Here's how the part is built. I have some questions about the finished solid (model axes, mm). A direction names the side the tool comes from. Coordinates: 2 decimals unless noted, no trailing zeros. Write each loop counter-clockwise with the first axis right and the second up, starting at its lowest first coordinate (ties: lowest second). Pieces come first, ordered by that corner, then holes.
Item 1: I'm going to push flat-ended pins straight in: P1, Ø3, axis at x = 13.97, z = -13.97, coming from the +Y side; P2, Ø10, axis at y = 16, z = -85, coming from the -X side; P3, Ø1, axis at y = 14.5, z = -32, coming from the -X side; P4, Ø5, axis at x = 14.5, z = -33.5, coming from the +Y side. Where does each tip first touch, or does it pass through?
Item 2: I want a section at B-B (z = -54). Please give me the cut outline in (x, y) (3 decimals).
Item 3: If we mould it in two halves opening along Z, with no side actions, what happens to faces 1 (the face through (9, 8, 0)), 2 (the face through (10, 0, -53)), 3 (the face through (6, 17, -81.661))? For each: pulls with the +Z half, pulls with the -Z half, needs draft (parallel to the pull), parting line crosses it, or undercut.
Item 4: Please list where these lines run through material, in increasing order: line 1 (Z direction, x = 13.97, y = 1.75); line 2 (X direction, y = 7.25, z = -96); line 3 (Y direction, x = 8.5, z = -78).
Item 5: I want a section at A-A (z = -13.97). Please give me the cut outline in (x, y) (3 decimals), and give its area (3 significant figures).
Item 6: For faces 4 (the face through (15, 2, -82.55)), 5 (the face through (7, 11.43, -111)), 6 (the face through (15, 3.048, -42)), 7 (the face through (1.29, 10.18, -110.81)), which set-ups out of +Z, -Z, +X, -X, +Y, -Y let a thin tool reach every point of the face, with its end or its side?
from build123d import *

# Parameters (mm, degrees)
SKETCH1_W           = 77.47
SKETCH1_H           = 133.35
BOSS_EXTRUDE1_DEPTH = 11.43
SKETCH2_R           = 3.429
CUT_EXTRUDE1_DEPTH  = 134.35
CUT_EXTRUDE2_DEPTH  = 12.43
SKETCH4_W           = 54.61
SKETCH4_H           = 6.35
CUT_EXTRUDE3_DEPTH  = 134.35
CHAMFER1_SIZE       = 2.54
CUT_EXTRUDE4_DEPTH  = 12.43
SKETCH6_W           = 53.34
SKETCH6_H           = 82.55
CUT_EXTRUDE5_DEPTH  = 12.43
SKETCH7_R           = 1.778
HOLE_CUTS_1_DEPTH   = 6.08
BOSS_EXTRUDE5_DEPTH = 88.9
SKETCH18_W          = 6.35
SKETCH18_H          = 5.08
CUT_EXTRUDE13_DEPTH = 76.2
HOLE_CUTS_2_REACH   = 10.608
SKETCH19_R          = 1.778
SKETCH20_W          = 88.9
SKETCH20_H          = 11.176
CUT_EXTRUDE16_DEPTH = 1.27
CUT_EXTRUDE22_DEPTH = 134.35
SKETCH22_W          = 6.35
SKETCH22_H          = 82.55
CUT_EXTRUDE18_DEPTH = 2.032
SKETCH23_W          = 1.676805636
SKETCH23_H          = 88.9
BOSS_EXTRUDE6_DEPTH = 1.27
CUT_EXTRUDE19_REACH = 10.019
SKETCH24_W          = 69.85
SKETCH24_H          = 9.3345
CUT_EXTRUDE20_REACH = 12.28
SKETCH25_W          = 1.27
SKETCH25_H          = 88.9
CUT_EXTRUDE21_REACH = 7.08
SKETCH26_W          = 6.35
SKETCH26_H          = 6.35


with BuildPart() as part:
    # Sketch1 → Boss-Extrude1 (new body)
    with BuildSketch(Plane(origin=(0, 0, 0), x_dir=(1, 0, 0), z_dir=(0, 1, 0))):
        with Locations((38.735, 66.675)):
            Rectangle(SKETCH1_W, SKETCH1_H)
    extrude(amount=BOSS_EXTRUDE1_DEPTH)

    # Sketch2 → Cut-Extrude1 (cut, through all)
    with BuildSketch(Plane.XY):
        with Locations((5.715, 5.715)):
            Circle(SKETCH2_R)
        with Locations((71.755, 5.715)):
            Circle(SKETCH2_R)
    extrude(amount=-CUT_EXTRUDE1_DEPTH, mode=Mode.SUBTRACT)

    # Sketch3 → Cut-Extrude2 (cut, through all)
    with BuildSketch(Plane(origin=(0, 11.43, 0), x_dir=(1, 0, 0), z_dir=(0, 1, 0))):
        with BuildLine():
            Line((11.43, 133.35), (11.43, 95.25))
            ThreePointArc((11.43, 95.25), (15.149743879, 86.269743879), (24.13, 82.55))
            Line((24.13, 82.55), (53.34, 82.55))
            ThreePointArc((53.34, 82.55), (62.320256121, 86.269743879), (66.04, 95.25))
            Line((66.04, 95.25), (66.04, 133.35))
            Line((66.04, 133.35), (11.43, 133.35))
        make_face()
    extrude(amount=-CUT_EXTRUDE2_DEPTH, mode=Mode.SUBTRACT)

    # Sketch4 → Cut-Extrude3 (cut, through all)
    with BuildSketch(Plane(origin=(0, 0, -133.35), x_dir=(-1, 0, 0), z_dir=(0, 0, -1))):
        with Locations((-38.735, 8.255)):
            Rectangle(SKETCH4_W, SKETCH4_H)
    extrude(amount=-CUT_EXTRUDE3_DEPTH, mode=Mode.SUBTRACT)

    # Chamfer1
    chamfer1_edges = [part.edges().sort_by_distance(p)[0] for p in [
        (77.47, 11.43, -66.675),
        (0, 11.43, -66.675),
        (77.47, 0, -66.675),
        (0, 0, -66.675),
    ]]
    chamfer(chamfer1_edges, length=CHAMFER1_SIZE)

    # Sketch5 → Cut-Extrude4 (cut, through all)
    with BuildSketch(Plane(origin=(0, 11.43, 0), x_dir=(1, 0, 0), z_dir=(0, 1, 0))):
        Polygon((11.43, 95.25), (11.43, 82.55), (77.47, 82.55), (77.47, 133.35), (11.43, 133.35), align=None)
    extrude(amount=-CUT_EXTRUDE4_DEPTH, mode=Mode.SUBTRACT)

    # Sketch6 → Cut-Extrude5 (cut, through all)
    with BuildSketch(Plane(origin=(0, 11.43, 0), x_dir=(1, 0, 0), z_dir=(0, 1, 0))):
        with Locations((50.8, 41.275)):
            Rectangle(SKETCH6_W, SKETCH6_H)
    extrude(amount=-CUT_EXTRUDE5_DEPTH, mode=Mode.SUBTRACT)

    # Sketch7 → Hole Cuts 1 (cut, through all)
    with BuildSketch(Plane(origin=(0, 5.08, 0), x_dir=(1, 0, 0), z_dir=(0, 1, 0))):
        with Locations((13.97, 74.93)):
            Circle(SKETCH7_R)
        with Locations((13.97, 13.97)):
            Circle(SKETCH7_R)
    extrude(amount=-HOLE_CUTS_1_DEPTH, mode=Mode.SUBTRACT)

    # Sketch17 → Boss-Extrude5 (add)
    with BuildSketch(Plane.XY):
        Polygon((0, 8.89), (0, 11.869940905), (5.588, 21.548640818), (8.851738686, 19.664320409), (5.930738686, 14.605), (11.43, 11.43), (2.54, 11.43), align=None)
    extrude(amount=-BOSS_EXTRUDE5_DEPTH)

    # Sketch18 → Cut-Extrude13 (cut)
    with BuildSketch(Plane.XY):
        with Locations((20.955, 2.54)):
            Rectangle(SKETCH18_W, SKETCH18_H)
    extrude(amount=-CUT_EXTRUDE13_DEPTH, mode=Mode.SUBTRACT)

    # Sketch19 → Hole Cuts 2 (cut, up to next)
    with BuildSketch(Plane(origin=(-1.876096497, 1.083164817, 0), x_dir=(0, 0, -1), z_dir=(0.866025404, -0.5, 0)), mode=Mode.PRIVATE) as hole_cuts_2_sk1:
        with Locations((8.382, 19.423670365)):
            Circle(SKETCH19_R)
    hole_cuts_2_tool1 = extrude(hole_cuts_2_sk1.sketch, amount=-HOLE_CUTS_2_REACH, mode=Mode.PRIVATE) & part.part
    add(hole_cuts_2_tool1.solids().sort_by_distance((7.835739, 17.904557, -8.382))[0], mode=Mode.SUBTRACT)
    # Sketch19 → Hole Cuts 2 (cut, up to next)
    with BuildSketch(Plane(origin=(-1.876096497, 1.083164817, 0), x_dir=(0, 0, -1), z_dir=(0.866025404, -0.5, 0)), mode=Mode.PRIVATE) as hole_cuts_2_sk2:
        with Locations((85.09, 19.423670365)):
            Circle(SKETCH19_R)
    hole_cuts_2_tool2 = extrude(hole_cuts_2_sk2.sketch, amount=-HOLE_CUTS_2_REACH, mode=Mode.PRIVATE) & part.part
    add(hole_cuts_2_tool2.solids().sort_by_distance((7.835739, 17.904557, -85.09))[0], mode=Mode.SUBTRACT)

    # Sketch20 → Cut-Extrude16 (cut)
    with BuildSketch(Plane(origin=(-5.139835183, 2.967485226, 0), x_dir=(0, 0, 1), z_dir=(-0.866025404, 0.5, 0))):
        with Locations((-44.45, 15.867670365)):
            Rectangle(SKETCH20_W, SKETCH20_H)
    extrude(amount=-CUT_EXTRUDE16_DEPTH, mode=Mode.SUBTRACT)

    # Sketch31 → Cut-Extrude22 (cut, through all)
    with BuildSketch(Plane.XY):
        Polygon((8.14000854, 20.075238), (12.539417591, 17.535238), (9.618417591, 12.475917591), (5.21900854, 15.015917591), align=None)
    extrude(amount=-CUT_EXTRUDE22_DEPTH, mode=Mode.SUBTRACT)

    # Sketch22 → Cut-Extrude18 (cut)
    with BuildSketch(Plane(origin=(0, 5.08, 0), x_dir=(1, 0, 0), z_dir=(0, 1, 0))):
        with Locations((14.605, 41.275)):
            Rectangle(SKETCH22_W, SKETCH22_H)
    extrude(amount=-CUT_EXTRUDE18_DEPTH, mode=Mode.SUBTRACT)

    # Sketch23 → Boss-Extrude6 (add)
    with BuildSketch(Plane(origin=(10.727835183, 18.581155592, 0), x_dir=(0.866025404, -0.5, 0), z_dir=(0.5, 0.866025404, 0))):
        with Locations((-3.826567635, 44.45)):
            Rectangle(SKETCH23_W, SKETCH23_H)
    extrude(amount=BOSS_EXTRUDE6_DEPTH)

    # Sketch24 → Cut-Extrude19 (cut, up to next)
    with BuildSketch(Plane(origin=(-2.587826643, 1.494082409, 0), x_dir=(0, 0, -1), z_dir=(0.866025404, -0.5, 0)), mode=Mode.PRIVATE) as cut_extrude19_sk1:
        with Locations((46.736, 18.058420365)):
            Rectangle(SKETCH24_W, SKETCH24_H)
    cut_extrude19_tool1 = extrude(cut_extrude19_sk1.sketch, amount=-CUT_EXTRUDE19_REACH, mode=Mode.PRIVATE) & part.part
    add(cut_extrude19_tool1.solids().sort_by_distance((6.441384, 17.133133, -46.736))[0], mode=Mode.SUBTRACT)

    # Sketch25 → Cut-Extrude20 (cut, up to next)
    with BuildSketch(Plane(origin=(5.139835183, 8.902455679, 0), x_dir=(0.866025404, -0.5, 0), z_dir=(0.5, 0.866025404, 0)), mode=Mode.PRIVATE) as cut_extrude20_sk1:
        with Locations((-5.299970453, 44.45)):
            Rectangle(SKETCH25_W, SKETCH25_H)
    cut_extrude20_tool1 = extrude(cut_extrude20_sk1.sketch, amount=-CUT_EXTRUDE20_REACH, mode=Mode.PRIVATE) & part.part
    add(cut_extrude20_tool1.solids().sort_by_distance((0.549926, 11.552441, -44.45))[0], mode=Mode.SUBTRACT)

    # Sketch26 → Cut-Extrude21 (cut, up to next)
    with BuildSketch(Plane(origin=(0, 5.08, 0), x_dir=(1, 0, 0), z_dir=(0, 1, 0)), mode=Mode.PRIVATE) as cut_extrude21_sk1:
        with Locations((20.955, 79.375)):
            Rectangle(SKETCH26_W, SKETCH26_H)
    cut_extrude21_tool1 = extrude(cut_extrude21_sk1.sketch, amount=-CUT_EXTRUDE21_REACH, mode=Mode.PRIVATE) & part.part
    add(cut_extrude21_tool1.solids().sort_by_distance((20.955, 5.08, -79.375))[0], mode=Mode.SUBTRACT)


solid = part.part
Answer:
1. P1: passes through
1. P2: stops at x = 0.96
1. P3: stops at x = 4.63
1. P4: stops at y = 3.05
2. outline: (0, 2.54) - (2.54, 0) - (17.78, 0) - (17.78, 3.048) - (11.43, 3.048) - (11.43, 11.43) - (5.219, 15.016) - (4.108, 13.091) - (2.656, 13.93) - (0, 9.33) - close; hole circle Ø6.858 at (5.715, 5.715)
3. face 1: pulls with the +Z half
3. face 2: needs draft
3. face 3: undercut
4. line 1: z = -82.55 to -76.71, -73.15 to -15.75, -12.19 to 0
4. line 2: x = 0 to 2.65, 8.78 to 11.43
4. line 3: y = 0 to 3.71, 7.72 to 13.12
5. outline: (0, 2.54) - (2.54, 0) - (12.192, 0) - (12.192, 3.048) - (11.43, 3.048) - (11.43, 11.43) - (5.219, 15.016) - (4.108, 13.091) - (2.656, 13.93) - (0, 9.33) - close; (15.748, 0) - (17.78, 0) - (17.78, 3.048) - (15.748, 3.048) - close; hole circle Ø6.858 at (5.715, 5.715)
5. area: 117 mm2
6. face 4: -Z, +X, +Y, -Y
6. face 5: -Z, +X, -X, +Y
6. face 6: +Z, -Z, +X, +Y
6. face 7: -Z, -X, +Y
